```python
from build123d import *

# Parameters (mm, degrees)
SKETCH1_W           = 44
SKETCH1_H           = 44
BOSS_EXTRUDE2_DEPTH = 2
SKETCH1_5_W         = 44
SKETCH1_5_H         = 44
SKETCH1_5_W_2       = 10
SKETCH1_5_H_2       = 10
BOSS_EXTRUDE3_DEPTH = 1


with BuildPart() as part:
    # Sketch1 → Boss-Extrude2 (new body)
    with BuildSketch(Plane(origin=(0, 0, 0), x_dir=(1, 0, 0), z_dir=(0, 1, 0))):
        with Locations((-7, -14)):
            Rectangle(SKETCH1_W, SKETCH1_H)
    extrude(amount=-BOSS_EXTRUDE2_DEPTH)

    # Sketch1_5 → Boss-Extrude3 (add)
    with BuildSketch(Plane(origin=(0, 0, 0), x_dir=(1, 0, 0), z_dir=(0, 1, 0))):
        with Locations((-7, -14)):
            Rectangle(SKETCH1_5_W, SKETCH1_5_H)
        with Locations((7, -28)):
            Rectangle(SKETCH1_5_W_2, SKETCH1_5_H_2, mode=Mode.SUBTRACT)
        with Locations((-21, -28)):
            Rectangle(SKETCH1_5_W_2, SKETCH1_5_H_2, mode=Mode.SUBTRACT)
        with Locations((-21, -14)):
            Rectangle(SKETCH1_5_W_2, SKETCH1_5_H_2, mode=Mode.SUBTRACT)
        with Locations((-7, -14)):
            Rectangle(SKETCH1_5_W_2, SKETCH1_5_H_2, mode=Mode.SUBTRACT)
        with Locations((-21, 0)):
            Rectangle(SKETCH1_5_W_2, SKETCH1_5_H_2, mode=Mode.SUBTRACT)
        with Locations((7, 0)):
            Rectangle(SKETCH1_5_W_2, SKETCH1_5_H_2, mode=Mode.SUBTRACT)
        with Locations((-7, 0)):
            Rectangle(SKETCH1_5_W_2, SKETCH1_5_H_2, mode=Mode.SUBTRACT)
        with Locations((-7, -28)):
            Rectangle(SKETCH1_5_W_2, SKETCH1_5_H_2, mode=Mode.SUBTRACT)
        with Locations((7, -14)):
            Rectangle(SKETCH1_5_W_2, SKETCH1_5_H_2, mode=Mode.SUBTRACT)
    extrude(amount=BOSS_EXTRUDE3_DEPTH)


solid = part.part
```
Input: part model. Units: mm. Frame: model coordinates. A direction names the side the tool comes from. Give positions to 0.01 mm unless a question says otherwise; leave off trailing zeros. Order: outer loops, then holes, each group sorted by start corner. A loop starts at its lowest first (then second) coordinate and runs counter-clockwise, first axis right, second up. Notation, with made-up numbers: M 41,85.5 L 74,85.5 A29 cw 74,118.5 Z; hole C -25.5,37.5 d10. An arc over 180 degrees is marked long. Return JSON: item names as keys, results as strings.
Item 1: Cut plane B-B (x = 9.5). Return loops of the section in (y, z), then the cut area to 3 significant figures.
Solutions:
{"outline": "M -2,-8 L 1,-8 L 1,-5 L 0,-5 L 0,5 L 1,5 L 1,9 L 0,9 L 0,19 L 1,19 L 1,23 L 0,23 L 0,33 L 1,33 L 1,36 L -2,36 Z", "area": "102 mm^2"}
Item 2: Ray query, probe 1 along Z at (x, y) = (-10.5, 0.2); probe 2 along X at (y, z) = (0.65, 3); probe 3 along Y at (x, z) = (7.5, 31). Return the intervals inside material, ascending.
Solutions:
{"probe 1": "-8 to -5, 5 to 9, 19 to 23, 33 to 36", "probe 2": "-29 to -26, -16 to -12, -2 to 2, 12 to 15", "probe 3": "-2 to 0"}
Item 3: First-contact query: P1, Ø3, axis at x = -18.5, z = 12.5, coming from the +Y side. Flat tip, straight axial feed; report the tip coordinate or a pass-through.
Solutions:
{"P1": "y = 0"}
Item 4: Pull-direction query (X, two-part tool) for faces 1 (the flat face through (-7, -1, -8)), 2 (the flat face through (-21.1, 0.5, 5)), 3 (the flat face through (15, -1, 14)); classes: +X half, -X half, draft (parallel to the pull), parting line (faces both ways), or undercut.
Solutions:
{"face 1": "draft", "face 2": "undercut", "face 3": "+X half"}
Item 5: Access query for faces 4 (the flat face through (-7.1, 0.5, 5)), 5 (the flat face through (-7, -1, 36)). Directions: +Z, -Z, +X, -X, +Y, -Y. A direction counts if a zero-diameter tool reaches every point of the face in a straight line with its end or side. Return the directions, or none.
Solutions:
{"face 4": "+Y", "face 5": "+Z, +X, -X, +Y, -Y"}
Item 6: Cut plane A-A (z = 28). Return loops of the section in (x, y).
Solutions:
{"outline": "M -29,-2 L 15,-2 L 15,1 L 12,1 L 12,0 L 2,0 L 2,1 L -2,1 L -2,0 L -12,0 L -12,1 L -16,1 L -16,0 L -26,0 L -26,1 L -29,1 Z"}
